```python
from build123d import *

# Parameters (mm, degrees)
SKETCH1_R           = 6.7818
BOSS_EXTRUDE1_DEPTH = 2.032
CHAMFER1_SIZE       = 1.016


with BuildPart() as part:
    # Sketch1 → Boss-Extrude1 (new, symmetric)
    with BuildSketch(Plane(origin=(0, 0, 0), x_dir=(1, 0, 0), z_dir=(0, 1, 0))):
        Polygon((6.833748726, 11.8364), (-6.833748726, 11.8364), (-13.667497452, 0), (-6.833748726, -11.8364), (6.833748726, -11.8364), (13.667497452, 0), align=None)
        with Locations(Location((0, 0, 0), (0, 0, 270))):
            Circle(SKETCH1_R, mode=Mode.SUBTRACT)
    extrude(amount=BOSS_EXTRUDE1_DEPTH, both=True)

    # Chamfer1
    chamfer1_edges = [part.edges().sort_by_distance(p)[0] for p in [
        (-10.250623089, 2.032, -5.9182),
        (-10.250623089, 2.032, 5.9182),
        (0, 2.032, 11.8364),
        (10.250623089, 2.032, 5.9182),
        (10.250623089, 2.032, -5.9182),
        (10.250623089, -2.032, 5.9182),
        (0, -2.032, 11.8364),
        (-10.250623089, -2.032, 5.9182),
        (-10.250623089, -2.032, -5.9182),
        (0, -2.032, -11.8364),
        (10.250623089, -2.032, -5.9182),
        (0, 2.032, -11.8364),
    ]]
    chamfer(chamfer1_edges, length=CHAMFER1_SIZE)


solid = part.part
```
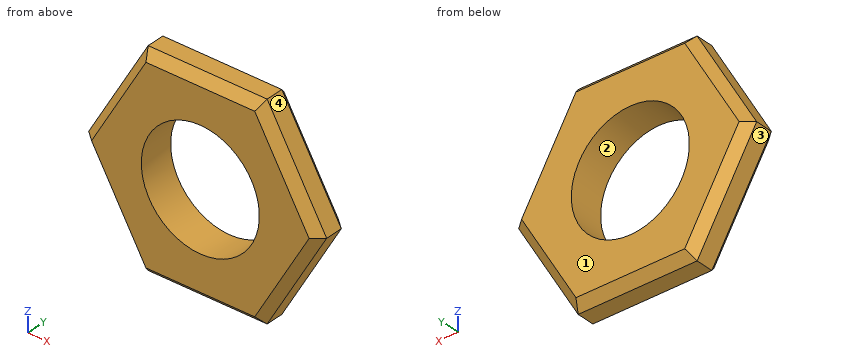
The model under review builds one solid part; all positions refer to its coordinate system, in mm. Face numbers are marked on the shaded views. Coordinates: 2 decimals unless noted, no trailing zeros. Write each loop counter-clockwise with the first axis right and the second up, starting at its lowest first coordinate (ties: lowest second). Pieces come first, ordered by that corner, then holes.
1) To check wall thickness, follow probe 1 along X at (y, z) = (-1.45, -1.25); probe 2 along X at (y, z) = (-0.45, -1); probe 3 along Z at (x, y) = (2.25, -1.25). State the ranges of each line that lie inside material, in increasing order.
2) We need section A-A on x = 0. State the section outline as (y, z) points.
3) We need section D-D on x = -8. State the section outline as (y, z) points.
4) The part is to be moulded in two halves that separate along X. For the marked faces 1, 2, 3 and 4, say which applies: pulls with the +X half, pulls with the -X half, needs draft (parallel to the pull), parting line crosses it, or undercut.
5) We need section B-B on y = 0. State the section outline as (x, z) points.
6) Clearance check with flat-ended pins moving along their axes: pin 1 Ø12 at (x, z) = (0, 0) entering from -Y; pin 2 Ø1 at (x, y) = (-10, 1) entering from +Z; pin 3 Ø1.5 at (x, y) = (-8, 1) entering from +Z. State where each tip first meets the part, or that it passes through.
7) We need section C-C on z = 2. State the section outline as (x, y) points.
Answer list:
1. probe 1: x = -12.44 to -6.67, 6.67 to 12.44
1. probe 2: x = -13.09 to -6.71, 6.71 to 13.09
1. probe 3: z = -11.6 to -6.4, 6.4 to 11.6
2. outline: (-2.03, -10.82) - (-1.02, -11.84) - (1.02, -11.84) - (2.03, -10.82) - (2.03, -6.78) - (-2.03, -6.78) - close; (-2.03, 6.78) - (2.03, 6.78) - (2.03, 10.82) - (1.02, 11.84) - (-1.02, 11.84) - (-2.03, 10.82) - close
3. outline: (-2.03, -7.78) - (-1.02, -9.82) - (1.02, -9.82) - (2.03, -7.78) - (2.03, 7.78) - (1.02, 9.82) - (-1.02, 9.82) - (-2.03, 7.78) - close
4. face 1: needs draft
4. face 2: undercut
4. face 3: pulls with the -X half
4. face 4: pulls with the +X half
5. outline: (-13.67, 0) - (-6.83, -11.84) - (6.83, -11.84) - (13.67, 0) - (6.83, 11.84) - (-6.83, 11.84) - close; hole circle Ø13.56 at (0, 0)
6. pin 1: passes through
6. pin 2: stops at z = 7.22
6. pin 3: stops at z = 11.12
7. outline: (-12.51, -1.02) - (-11.34, -2.03) - (-6.48, -2.03) - (-6.48, 2.03) - (-11.34, 2.03) - (-12.51, 1.02) - close; (6.48, -2.03) - (11.34, -2.03) - (12.51, -1.02) - (12.51, 1.02) - (11.34, 2.03) - (6.48, 2.03) - close
